from build123d import *

# Parameters (mm, degrees)
SKETCH2_W           = 50
SKETCH2_H           = 30
SKETCH2_W_2         = 42
SKETCH2_H_2         = 22
BOSS_EXTRUDE1_DEPTH = 28.8
SKETCH3_W           = 50
SKETCH3_H           = 30
BOSS_EXTRUDE2_DEPTH = 4
SKETCH4_W           = 22
SKETCH4_H           = 17.8
CUT_EXTRUDE1_DEPTH  = 4
SKETCH5_W           = 30
SKETCH5_H           = 32.8
BOSS_EXTRUDE3_DEPTH = 4
BOSS_EXTRUDE4_DEPTH = 4
SKETCH7_R           = 0.875
CUT_EXTRUDE2_DEPTH  = 10
SKETCH8_R           = 0.875
BOSS_EXTRUDE5_DEPTH = 4
FILLET1_R           = 3
BOSS_EXTRUDE6_START = -5
SKETCH9_R           = 0.875
BOSS_EXTRUDE6_DEPTH = 5
FILLET2_R           = 1
SKETCH11_R          = 0.875
SKETCH11_W          = 42
SKETCH11_H          = 22
BOSS_EXTRUDE7_DEPTH = 1
SKETCH14_R          = 5
CUT_EXTRUDE3_DEPTH  = 37
SKETCH17_R          = 7.5
CUT_EXTRUDE4_DEPTH  = 57.873262079
SKETCH18_R          = 5
BOSS_EXTRUDE9_DEPTH = 4
CUT_EXTRUDE5_DEPTH  = 75.343138703


with BuildPart() as part:
    # Sketch2 → Boss-Extrude1 (new body)
    with BuildSketch(Plane(origin=(0, 0, 0), x_dir=(1, 0, 0), z_dir=(0, 1, 0))):
        Rectangle(SKETCH2_W, SKETCH2_H)
        Rectangle(SKETCH2_W_2, SKETCH2_H_2, mode=Mode.SUBTRACT)
    extrude(amount=BOSS_EXTRUDE1_DEPTH)

    # Sketch3 → Boss-Extrude2 (add)
    with BuildSketch(Plane.XZ):
        Rectangle(SKETCH3_W, SKETCH3_H)
    extrude(amount=BOSS_EXTRUDE2_DEPTH)

    # Sketch4 → Cut-Extrude1 (cut)
    with BuildSketch(Plane(origin=(25, 0, 0), x_dir=(0, 0, -1), z_dir=(1, 0, 0))):
        with Locations((0, 4.9)):
            Rectangle(SKETCH4_W, SKETCH4_H)
    extrude(amount=-CUT_EXTRUDE1_DEPTH, mode=Mode.SUBTRACT)

    # Sketch5 → Boss-Extrude3 (add)
    with BuildSketch(Plane.ZY.offset(25)):
        with Locations((0, 12.4)):
            Rectangle(SKETCH5_W, SKETCH5_H)
    extrude(amount=BOSS_EXTRUDE3_DEPTH)

    # Sketch6 → Boss-Extrude4 (add)
    with BuildSketch(Plane(origin=(25, 0, 0), x_dir=(0, 0, -1), z_dir=(1, 0, 0))):
        Polygon((-15, -4), (-11, -4), (-11, 13.8), (11, 13.8), (11, -4), (15, -4), (15, 28.8), (-15, 28.8), align=None)
    extrude(amount=BOSS_EXTRUDE4_DEPTH)

    # Sketch7 → Cut-Extrude2 (cut)
    with BuildSketch(Plane(origin=(0, 28.8, 0), x_dir=(1, 0, 0), z_dir=(0, 1, 0))):
        with Locations(Location((23, -5, 0), (0, 0, 270))):
            Circle(SKETCH7_R)
        with Locations(Location((23, 5, 0), (0, 0, 270))):
            Circle(SKETCH7_R)
        with Locations(Location((-25, 5, 0), (0, 0, 270))):
            Circle(SKETCH7_R)
        with Locations(Location((-25, -5, 0), (0, 0, 270))):
            Circle(SKETCH7_R)
    extrude(amount=-CUT_EXTRUDE2_DEPTH, mode=Mode.SUBTRACT)

    # Sketch8 → Boss-Extrude5 (add)
    with BuildSketch(Plane.XZ.offset(4)):
        with BuildLine():
            Line((20.903006959, -15), (30.229257675, -15))
            ThreePointArc((30.229257675, -15), (32.740161395, -15.676186578), (34.571929358, -17.521854998))
            ThreePointArc((34.571929358, -17.521854998), (40.295729423, -19.918118011), (44.079388874, -15))
            Line((44.079388874, -15), (44.079388874, 15))
            ThreePointArc((44.079388874, 15), (40.295729423, 19.918118011), (34.571929358, 17.521854998))
            ThreePointArc((34.571929358, 17.521854998), (32.740161395, 15.676186578), (30.229257675, 15))
            Line((30.229257675, 15), (20.903006959, 15))
            Line((20.903006959, 15), (20.903006959, -15))
        make_face()
        with Locations(Location((38.991197916, 15, 0), (0, 0, 270))):
            Circle(SKETCH8_R, mode=Mode.SUBTRACT)
        with Locations(Location((38.991197916, -15, 0), (0, 0, 270))):
            Circle(SKETCH8_R, mode=Mode.SUBTRACT)
    extrude(amount=-BOSS_EXTRUDE5_DEPTH)

    # Fillet1
    fillet1_edges = [part.edges().sort_by_distance(p)[0] for p in [
        (29, 0, -13),
        (29, 0, 13),
    ]]
    fillet(fillet1_edges, radius=FILLET1_R)

    # Sketch9 → Boss-Extrude6 (add)
    with BuildSketch(Plane(origin=(0, 28.8, 0), x_dir=(1, 0, 0), z_dir=(0, 1, 0)).offset(BOSS_EXTRUDE6_START)):
        with BuildLine():
            Line((30.229257675, 15), (26.332891716, 15))
            Line((26.332891716, 15), (26.332891716, -15))
            Line((26.332891716, -15), (30.229257675, -15))
            ThreePointArc((30.229257675, -15), (31.129332579, -15.081680656), (32, -15.324053934))
            ThreePointArc((32, -15.324053934), (33.477494133, -16.198821247), (34.571929358, -17.521854998))
            ThreePointArc((34.571929358, -17.521854998), (40.295729423, -19.918118011), (44.079388874, -15))
            Line((44.079388874, -15), (44.079388874, 15))
            ThreePointArc((44.079388874, 15), (40.295729423, 19.918118011), (34.571929358, 17.521854998))
            ThreePointArc((34.571929358, 17.521854998), (33.477494133, 16.198821247), (32, 15.324053934))
            ThreePointArc((32, 15.324053934), (31.129332579, 15.081680656), (30.229257675, 15))
        make_face()
        with Locations(Location((38.991197916, -15, 0), (0, 0, 90))):
            Circle(SKETCH9_R, mode=Mode.SUBTRACT)
        with Locations(Location((38.991197916, 15, 0), (0, 0, 90))):
            Circle(SKETCH9_R, mode=Mode.SUBTRACT)
    extrude(amount=BOSS_EXTRUDE6_DEPTH)

    # Fillet2
    fillet2_edges = [part.edges().sort_by_distance(p)[0] for p in [
        (29, 23.8, 0),
    ]]
    fillet(fillet2_edges, radius=FILLET2_R)

    # Sketch11 → Boss-Extrude7 (add)
    with BuildSketch(Plane(origin=(0, 28.8, 0), x_dir=(1, 0, 0), z_dir=(0, 1, 0))):
        with BuildLine():
            Line((-29, -15), (30.229257675, -15))
            ThreePointArc((30.229257675, -15), (32.740161395, -15.676186578), (34.571929358, -17.521854998))
            ThreePointArc((34.571929358, -17.521854998), (40.295729423, -19.918118011), (44.079388874, -15))
            Line((44.079388874, -15), (44.079388874, 15))
            ThreePointArc((44.079388874, 15), (40.295729423, 19.918118011), (34.571929358, 17.521854998))
            ThreePointArc((34.571929358, 17.521854998), (32.740161395, 15.676186578), (30.229257675, 15))
            Line((30.229257675, 15), (-29, 15))
            Line((-29, 15), (-29, -15))
        make_face()
        with Locations(Location((-25, 5, 0), (0, 0, 270))):
            Circle(SKETCH11_R, mode=Mode.SUBTRACT)
        with Locations(Location((-25, -5, 0), (0, 0, 270))):
            Circle(SKETCH11_R, mode=Mode.SUBTRACT)
        with Locations(Location((23, 5, 0), (0, 0, 270))):
            Circle(SKETCH11_R, mode=Mode.SUBTRACT)
        with Locations(Location((23, -5, 0), (0, 0, 270))):
            Circle(SKETCH11_R, mode=Mode.SUBTRACT)
        with Locations(Location((38.991197916, -15, 0), (0, 0, 90))):
            Circle(SKETCH11_R, mode=Mode.SUBTRACT)
        with Locations(Location((38.991197916, 15, 0), (0, 0, 90))):
            Circle(SKETCH11_R, mode=Mode.SUBTRACT)
        Rectangle(SKETCH11_W, SKETCH11_H, mode=Mode.SUBTRACT)
    extrude(amount=BOSS_EXTRUDE7_DEPTH)

    # Sketch14 → Cut-Extrude3 (cut)
    with BuildSketch(Plane.XZ.offset(4)):
        with Locations(Location((10.09, 0, 0), (0, 0, 270))):
            Circle(SKETCH14_R)
    extrude(amount=-CUT_EXTRUDE3_DEPTH, mode=Mode.SUBTRACT)

    # Sketch17 → Cut-Extrude4 (cut, through all)
    with BuildSketch(Plane(origin=(0, 0, 0), x_dir=(1, 0, 0), z_dir=(0, 1, 0))):
        with Locations(Location((-10.09, 0, 0), (0, 0, 90))):
            Circle(SKETCH17_R)
    extrude(amount=-CUT_EXTRUDE4_DEPTH, mode=Mode.SUBTRACT)

    # Sketch18 → Boss-Extrude9 (add)
    with BuildSketch(Plane.XZ.offset(4)):
        with Locations((10.09, 0)):
            Circle(SKETCH18_R)
    extrude(amount=-BOSS_EXTRUDE9_DEPTH)

    # Sketch19 → Cut-Extrude5 (cut, through all)
    with BuildSketch(Plane(origin=(-21, 0, 0), x_dir=(0, 0, -1), z_dir=(1, 0, 0))):
        Polygon((-11, 13.8), (11, 13.8), (11, 0), (-11, 0), (-11, 3), align=None)
    extrude(amount=-CUT_EXTRUDE5_DEPTH, mode=Mode.SUBTRACT)


solid = part.part
Read the model definition and answer for the solid it produces. Units are mm, in the model's axes. A direction names the side the tool comes from. Coordinates: 2 decimals unless noted, no trailing zeros. Loops run counter-clockwise (first coordinate to the right, second up) from the corner with the lowest first, then second, coordinate; pieces in that order, holes last.
Q1. The mould has two halves that part along Y. Classify faces 6 (the face through (2, 15, -11)), 7 (the face through (39.845, 26.758, -14.81)): +Y half, -Y half, draft (parallel to the pull), parting line (faces both ways), or undercut.
Q2. The part is cut by section D-D on x = -3.5. Write down the section's boundary in (y, z).
Q3. Each of these flat-tipped pins is pushed along its axis until it touches: pin 1 Ø3 at (x, y) = (-17.5, 11) entering from -Z; pin 2 Ø1.6 at (x, z) = (23, -5) entering from +Y; pin 3 Ø2 at (x, y) = (17, 7.5) entering from +Z; pin 4 Ø1.1 at (x, z) = (38.99, -15) entering from +Y. Where does it stop, or does it pass through?
Q4. Which of the six approach directions +Z, -Z, +X, -X, +Y, -Y give full straight-line access (tool end or side, diameter ignored) to faces 1 (the face through (29.9, 0.86, -13.19)), 2 (the face through (1, 13, -15)), 3 (the face through (-25, 13.8, 0)), 4 (the face through (22.146, 24.223, 4.81)), 5 (the face through (2, 15, 11))?
Q5. Consider probe 1 along X at (y, z) = (21.5, -5) (3 decimals); probe 2 along Z at (x, y) = (10, 11.5); probe 3 along Y at (x, z) = (37, 14.5). Determine where each line is inside the solid, lowest interval first.
Q6. The part is cut by section B-B on z = -9. Write down the section's boundary in (x, y), and give its area (3 significant figures).
Q7. The part is cut by section A-A on y = 7. Write down the section's boundary in (x, z), and give its area (3 significant figures).
Q8. The part is cut by section C-C on z = 0. Write down the section's boundary in (x, y), and give its area (3 significant figures).
Results below:
1. face 6: undercut
1. face 7: draft
2. outline: (-4, -15) - (29.8, -15) - (29.8, -11) - (0, -11) - (0, -3.58) - (-4, -3.58) - close; (-4, 3.58) - (0, 3.58) - (0, 11) - (29.8, 11) - (29.8, 15) - (-4, 15) - close
3. pin 1: stops at z = -15
3. pin 2: stops at y = 18.8
3. pin 3: stops at z = 15
3. pin 4: passes through
4. face 1: +Z, -Z, +X
4. face 2: -Z, -X, +Y, -Y
4. face 3: +X, -X
4. face 4: +Y
4. face 5: none
5. probe 1: x = -29 to -25.875, -24.125 to -21, 21 to 22.125, 23.875 to 29
5. probe 2: z = -15 to -11, 11 to 15
5. probe 3: y = -4 to 0, 23.8 to 29.8
6. outline: (-29, -4) - (44.08, -4) - (44.08, 0) - (-29, 0) - close; (-29, 13.8) - (-21, 13.8) - (-21, 29.8) - (-29, 29.8) - close; (21, 13.8) - (29, 13.8) - (29, 22.8) arc R1 cw to (30, 23.8) - (44.08, 23.8) - (44.08, 29.8) - (21, 29.8) - close
6. area: 639 mm2
7. outline: (-29, -15) - (29, -15) - (29, -11) - (-29, -11) - close; (-29, 11) - (29, 11) - (29, 15) - (-29, 15) - close
7. area: 464 mm2
8. outline: (-29, -4) - (-17.59, -4) - (-17.59, 0) - (-29, 0) - close; (-29, 13.8) - (-21, 13.8) - (-21, 29.8) - (-29, 29.8) - close; (-2.59, -4) - (44.08, -4) - (44.08, 0) - (-2.59, 0) - close; (21, 13.8) - (29, 13.8) - (29, 22.8) arc R1 cw to (30, 23.8) - (44.08, 23.8) - (44.08, 29.8) - (21, 29.8) - close
8. area: 579 mm2
